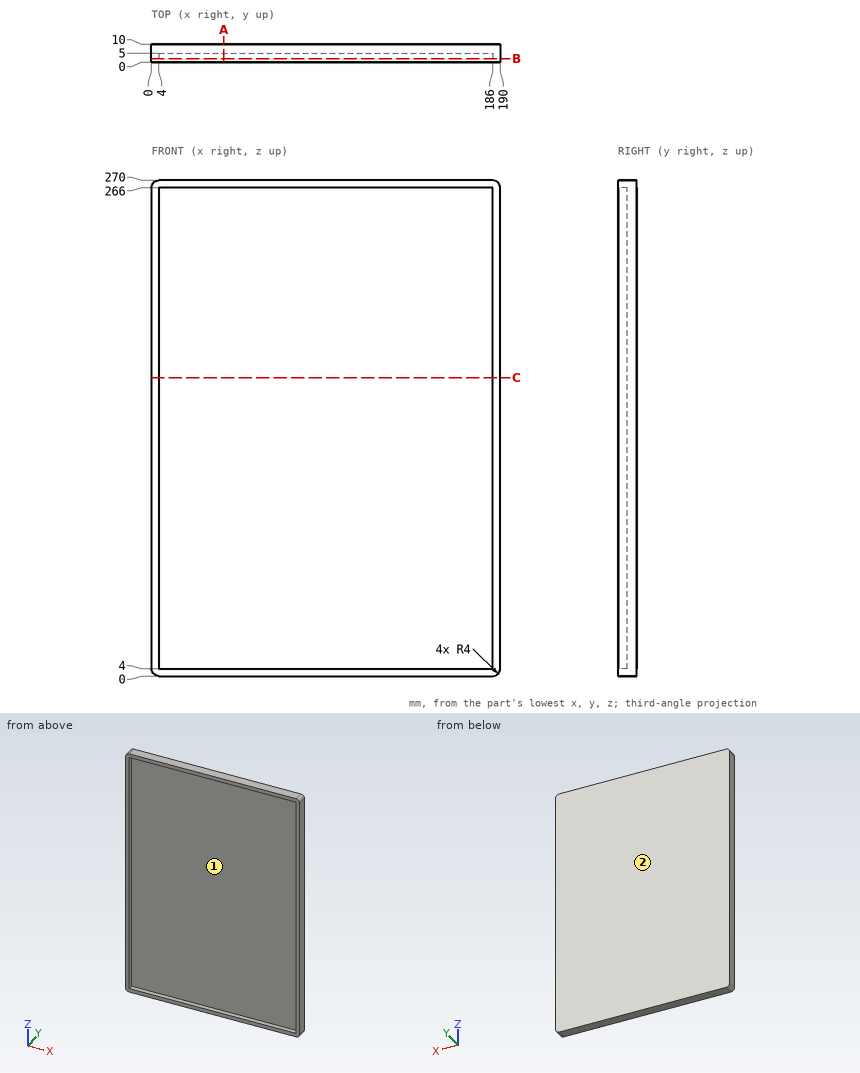
The figure shows three views and two pictorial views of one solid part (mm, origin at its lowest corner). Answer the questions. Give positions to 0.01 mm unless a question says otherwise; leave off trailing zeros. Loops run counter-clockwise (first coordinate to the right, second up) from the corner with the lowest first, then second, coordinate; pieces in that order, holes last. Notation, with made-up numbers: (-29, 41) -> (4, 41) arc R13 cw to (4, 47) -> close; hole circle Ø5 at (25, -26.5). An arc over 180 degrees is marked (long way). Put each result on its own line as item: value. Start each with the question number.
Item 1: This flat-tipped pin is pushed along its axis until it touches: P1, Ø1, axis at x = 120, z = 137, coming from the -Y side. Where does it stop, or does it pass through?
Item 2: The part is cut by section C-C (z = 162.5). Give the vertices of the cut face in (x, y), then the cut area to 3 significant figures.
Item 3: The part is cut by section B-B (y = 2). Give the vertices of the cut face in (x, z).
Item 4: Find the intervals of material crossed by L1, parallel to X at y = 0.5, z = 118.5; L2, parallel to Z at x = 102, y = 0.5; L3, parallel to Y at x = 14, z = 63, in increasing order. Write a range as [from, to].
Item 5: The part is cut by section A-A (x = 39.5). Give the vertices of the cut face in (y, z), then the cut area to 3 significant figures.
Item 6: The mould has two halves that part along Z. Classify the marked faces 1 and 2: released by +Z, released by -Z, zero draft, split by the parting line, or undercut.
Answers below:
1. P1: y = 5
2. outline: (0, 0) -> (4, 0) -> (4, 5) -> (186, 5) -> (186, 0) -> (190, 0) -> (190, 10) -> (0, 10) -> close
2. area: 990 mm2
3. outline: (0, 4) arc R4 ccw to (4, 0) -> (186, 0) arc R4 ccw to (190, 4) -> (190, 266) arc R4 ccw to (186, 270) -> (4, 270) arc R4 ccw to (0, 266) -> close; hole (4, 4) -> (186, 4) -> (186, 266) -> (4, 266) -> close
4. L1: [0, 4], [186, 190]
4. L2: [0, 4], [266, 270]
4. L3: [5, 10]
5. outline: (0, 0) -> (10, 0) -> (10, 270) -> (0, 270) -> (0, 266) -> (5, 266) -> (5, 4) -> (0, 4) -> close
5. area: 1,390 mm2
6. face 1: undercut
6. face 2: zero draft
